Geometry: see drawing. Coordinates: mm, zero at the bounding-box minimum. A direction names the side the tool comes from. Give positions to 0.01 mm unless a question says otherwise; leave off trailing zeros. Order: outer loops, then holes, each group sorted by start corner. A loop starts at its lowest first (then second) coordinate and runs counter-clockwise, first axis right, second up. Notation, with made-up numbers: (46.25, 45.5) - (82.25, 45.5) arc R17 cw to (82.25, 63.5) - close; hole circle Ø4 at (89, 39.5). An arc over 180 degrees is marked (long way). One line per item, written item: value.
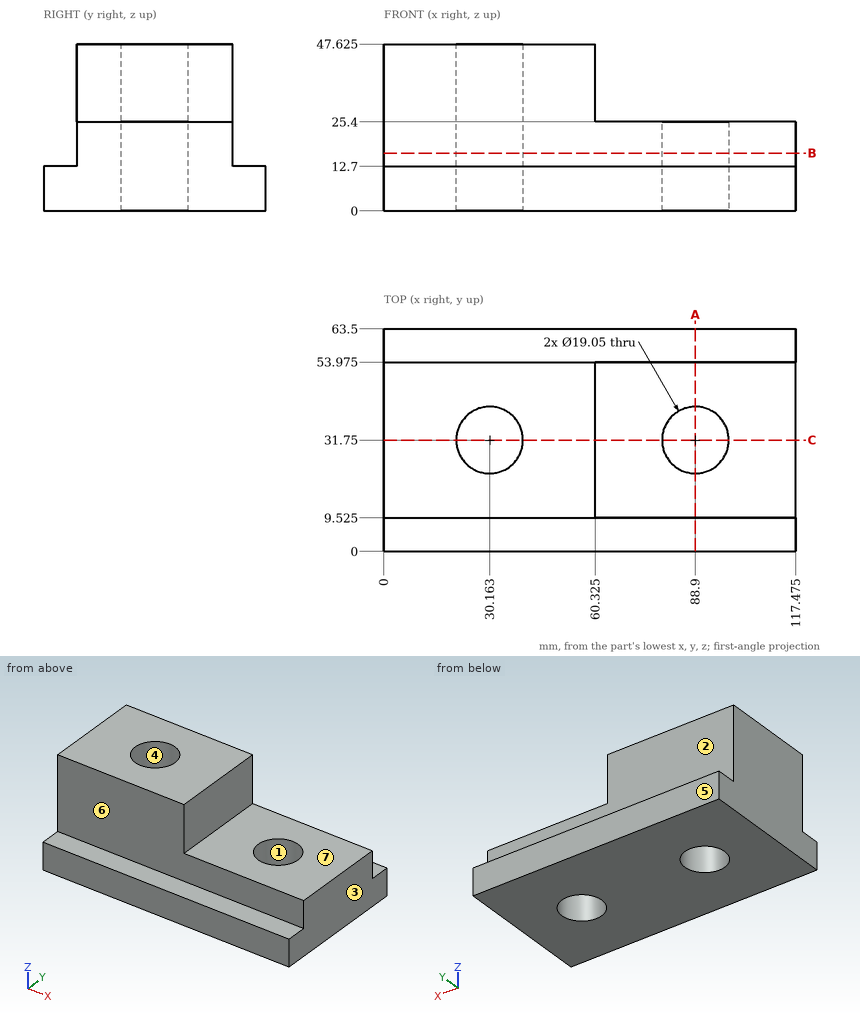
1) Set-up query: the marked faces 5, 6 and 7. Return all of +Z, -Z, +X, -X, +Y, -Y with unobstructed straight access to the full face (end or side cutting, diameter ignored); none if empty.
Answers below:
face 5: +Z, -Z, +X, -X, +Y
face 6: +Z, +X, -X, -Y
face 7: +Z, +X, +Y, -Y
2) Material intervals for line 1 along X through (y, z) = (29, 19.5) (1 decimal); line 2 along X through (y, z) = (33, 14.5) (1 decimal); line 3 along Y through (x, z) = (58.5, 31) (1 decimal), sorted ascending.
Answers below:
line 1: 0 to 21, 39.3 to 79.8, 98 to 117.5
line 2: 0 to 20.7, 39.6 to 79.5, 98.3 to 117.5
line 3: 9.5 to 54
3) Section C-C, the plane y = 31.75. Return loops of the section in (x, z) (1 decimal), then the cut area to 3 significant figures.
Answers below:
outline: (0, 0) - (20.6, 0) - (20.6, 47.6) - (0, 47.6) - close; (39.7, 0) - (79.4, 0) - (79.4, 25.4) - (60.3, 25.4) - (60.3, 47.6) - (39.7, 47.6) - close; (98.4, 0) - (117.5, 0) - (117.5, 25.4) - (98.4, 25.4) - close
area: 2,930 mm^2
4) First-contact query: pin 1 (2 mm diameter, centred on y = 25, z = 30.5, fed in from +X) (1 decimal); pin 2 (17.5 mm diameter, centred on x = 40.5, z = 37, fed in from -Y) (1 decimal); pin 3 (7.5 mm diameter, centred on x = 83, y = 4, fed in from +Z). Flat tips, straight axial feed; report the tip coordinate or a pass-through.
Answers below:
pin 1: x = 60.3
pin 2: y = 9.5
pin 3: z = 12.7
5) Section B-B, the plane z = 16.5. Count the separate pieces of the cut face and the enclosed holes in it, then the cut area to 3 significant figures.
Answers below:
separate pieces: 1
enclosed holes: 2
area: 4,650 mm^2
6) Section A-A, the plane x = 88.9. Return loops of the section in (y, z) (1 decimal).
Answers below:
outline: (0, 0) - (22.2, 0) - (22.2, 25.4) - (9.5, 25.4) - (9.5, 12.7) - (0, 12.7) - close; (41.3, 0) - (63.5, 0) - (63.5, 12.7) - (54, 12.7) - (54, 25.4) - (41.3, 25.4) - close
7) Mould query, pull axis X, two halves, no side actions, for the marked faces 1, 2, 3 and 4. Classes: released by +X, released by -X, zero draft, split by the parting line, or undercut.
Answers below:
face 1: undercut
face 2: zero draft
face 3: released by +X
face 4: undercut
